Check sheet for the drawn part. Datum: minimum x, y, z corner. Units: mm. Round coordinates to 2 decimals unless told otherwise and drop trailing zeros. Write each loop counter-clockwise with the first axis right and the second up, starting at its lowest first coordinate (ties: lowest second). Pieces come first, ordered by that corner, then holes. Notation, with made-up numbers: M 25.25,49.25 L 80.25,49.25 A14 cw 80.25,64.25 Z; hole C 49,3.5 d4. An arc over 180 degrees is marked long. One line per item, written item: value.
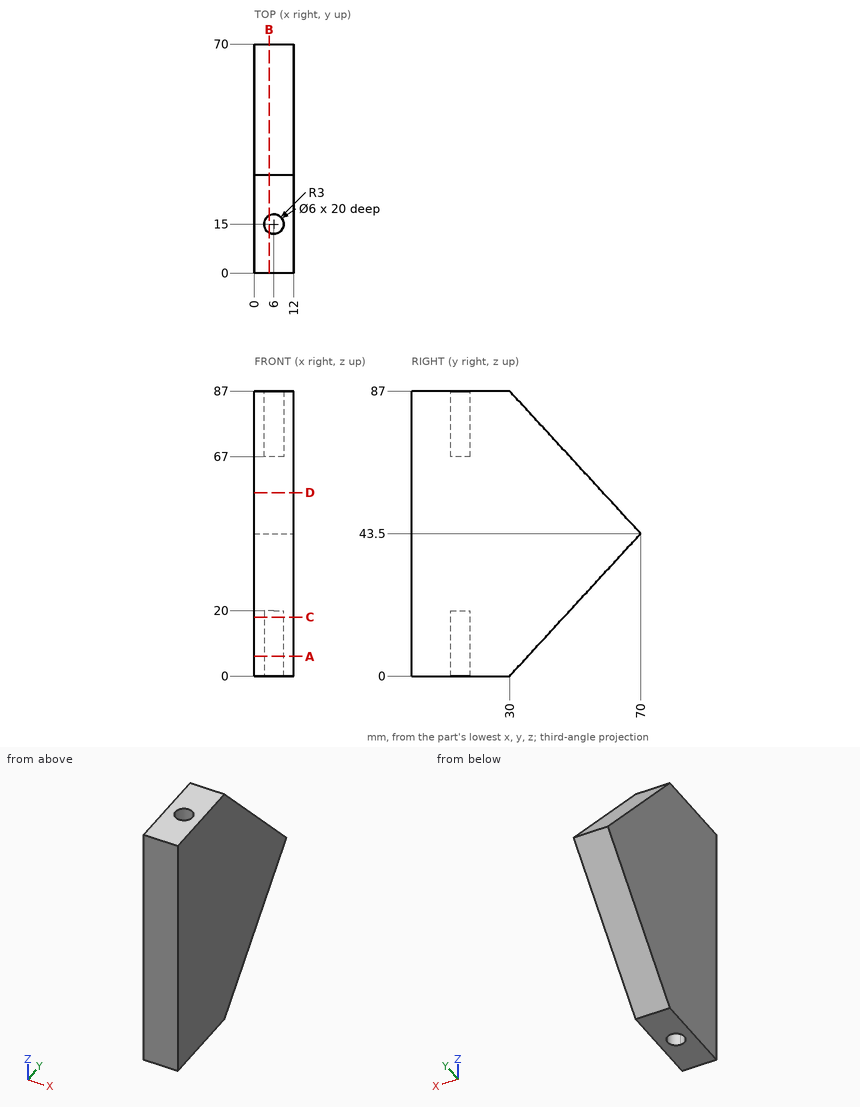
Q1. Depth check by flat-ended pin: P1, Ø5, axis at y = 26.5, z = 35.5, coming from the -X side; P2, Ø3, axis at x = 8.5, z = 31, coming from the +Y side; P3, Ø3, axis at x = 7.5, y = 40.5, coming from the +Z side; P4, Ø1.8, axis at x = 5.5, y = 16, coming from the +Z side. Enter the tip coordinate at first touch or a pass-through.
Completed:
P1: x = 0
P2: y = 59.89
P3: z = 77.21
P4: z = 67
Q2. Scan lines: line 1 (X direction, y = 13.5, z = 9.5); line 2 (Y direction, x = 6, z = 71.75); line 3 (Y direction, x = 6, z = 83.25). Record each from-to range of solid material in increasing order. Write a range as [from, to].
Completed:
line 1: [0, 3.4], [8.6, 12]
line 2: [0, 12], [18, 44.02]
line 3: [0, 12], [18, 33.45]
Q3. Sectioned sample at C-C on z = 18. Enter the section's corners in (x, y).
Completed:
outline: M 0,0 L 12,0 L 12,46.55 L 0,46.55 Z; hole M 6,12 A3 ccw 9,15 A3 ccw 6,18 A3 ccw Z
Q4. Sectioned sample at B-B on x = 4.5. Enter the section's corners in (y, z).
Completed:
outline: M 0,0 L 12.4,0 L 12.4,20 L 17.6,20 L 17.6,0 L 30,0 L 70,43.5 L 30,87 L 17.6,87 L 17.6,67 L 12.4,67 L 12.4,87 L 0,87 Z
Q5. Sectioned sample at D-D on z = 56. Enter the section's corners in (x, y), and give its area (3 significant figures).
Completed:
outline: M 0,0 L 12,0 L 12,58.51 L 0,58.51 Z
area: 702 mm^2
Q6. Sectioned sample at A-A on z = 6. Enter the section's corners in (x, y), and give its area (3 significant figures).
Completed:
outline: M 0,0 L 12,0 L 12,35.52 L 0,35.52 Z; hole M 6,12 A3 ccw 9,15 A3 ccw 6,18 A3 ccw Z
area: 398 mm^2
